```python
from build123d import *

# Parameters (mm, degrees)
SKETCH1_W                                      = 38.1
SKETCH1_H                                      = 127
BOSS_EXTRUDE1_DEPTH                            = 6.35
CBORE_FOR_4_SOCKET_HEAD_CAP_SCREW1_D           = 3.2639
CBORE_FOR_4_SOCKET_HEAD_CAP_SCREW1_CBORE_D     = 5.55752
CBORE_FOR_4_SOCKET_HEAD_CAP_SCREW1_CBORE_DEPTH = 2.8448


with BuildPart() as part:
    # Sketch1 → Boss-Extrude1 (new body)
    with BuildSketch(Plane(origin=(0, 0, 0), x_dir=(1, 0, 0), z_dir=(0, 1, 0))):
        Rectangle(SKETCH1_W, SKETCH1_H)
    extrude(amount=BOSS_EXTRUDE1_DEPTH)

    # CBORE for #4 Socket Head Cap Screw1 (through all)
    with Locations(Plane(origin=(0, 6.35, 0), x_dir=(1, 0, 0), z_dir=(0, 1, 0))):
        with Locations((-15.875, -57.15), (-15.875, 57.15)):
            CounterBoreHole(CBORE_FOR_4_SOCKET_HEAD_CAP_SCREW1_D / 2, CBORE_FOR_4_SOCKET_HEAD_CAP_SCREW1_CBORE_D / 2, CBORE_FOR_4_SOCKET_HEAD_CAP_SCREW1_CBORE_DEPTH)


solid = part.part
```
Source: CAD feature listing. Evaluate the final solid. Frame: model axes, mm. A direction names the side the tool comes from. Give positions to 0.01 mm unless a question says otherwise; leave off trailing zeros. Write each loop counter-clockwise with the first axis right and the second up, starting at its lowest first coordinate (ties: lowest second). Pieces come first, ordered by that corner, then holes.
1. First-contact query: pin 1 (3.5 mm diameter, centred on x = -15.875, z = -57.15, fed in from +Y). Flat tip, straight axial feed; report the tip coordinate or a pass-through.
2. Section query A-A (z = -57.15). Return the cut outline in (x, y), then the cut area to 3 significant figures.
3. Material intervals for line 1 along X through (y, z) = (1.05, 57.15); line 2 along X through (y, z) = (5.1, 57.15), sorted ascending.
4. Access query for faces 1 (the face through (-17.92, 4.95, -59.03)), 2 (the face through (19.05, 3, 1)). Directions: +Z, -Z, +X, -X, +Y, -Y. A direction counts if a zero-diameter tool reaches every point of the face in a straight line with its end or side. Return the directions, or none.
5. Pull-direction query (Z, two-part tool) for faces 3 (the face through (0, 6.35, -1)), 4 (the face through (-18.08, 4.95, 58.84)), 5 (the face through (0, 3, 63.5)), 6 (the face through (0, 3, -63.5)); classes: +Z half, -Z half, draft (parallel to the pull), parting line (faces both ways), or undercut.
Output values:
1. pin 1: stops at y = 3.51
2. outline: (-19.05, 0) - (-17.51, 0) - (-17.51, 3.51) - (-18.65, 3.51) - (-18.65, 6.35) - (-19.05, 6.35) - close; (-14.24, 0) - (19.05, 0) - (19.05, 6.35) - (-13.1, 6.35) - (-13.1, 3.51) - (-14.24, 3.51) - close
2. area: 215 mm2
3. line 1: x = -19.05 to -17.51, -14.24 to 19.05
3. line 2: x = -19.05 to -18.65, -13.1 to 19.05
4. face 1: +Y
4. face 2: +Z, -Z, +X, +Y, -Y
5. face 3: draft
5. face 4: undercut
5. face 5: +Z half
5. face 6: -Z half
